Read the model definition and answer for the solid it produces. Units are mm, in the model's axes. A direction names the side the tool comes from. Coordinates: 2 decimals unless noted, no trailing zeros. Write each loop counter-clockwise with the first axis right and the second up, starting at its lowest first coordinate (ties: lowest second). Pieces come first, ordered by that corner, then holes. Notation, with made-up numbers: (34, 85) -> (39, 85) arc R32 ccw to (39, 116) -> close; hole circle Ø1 at (33, 86). An arc over 180 degrees is marked (long way). Use CSV: the item, a comma, the result in double quotes.
Autodesk Inventor part; units mm, degrees
ref_plane "YZ Plane" through (0, 0, 0) normal (1, 0, 0) x (0, 1, 0)
ref_plane "XZ Plane" through (0, 0, 0) normal (0, 1, 0) x (-1, 0, 0)
ref_plane "XY Plane" through (0, 0, 0) normal (0, 0, 1) x (1, 0, 0)
sketch "Sketch1" plane through (0, 0, 0) normal (0, 0, 1) x (1, 0, 0)
  circle A0 centre (0, 0) radius 22.225
  circle A1 centre (0, 0) radius 28.575
  line L0 (0, 0) -> (-22.225, 0) construction
  line L1 (-26.1937, 1.5875) -> (-24.6062, 1.5875)
  line L2 (-24.6062, 1.5875) -> (-24.6062, -1.5875)
  line L3 (-24.6062, -1.5875) -> (-26.1937, -1.5875)
  line L4 (-26.1937, -1.5875) -> (-26.1937, 1.5875)
  line L5 (-22.225, 0) -> (-28.575, 0) construction
  line L6 (-25.4, 1.5875) -> (-25.4, -1.5875) construction
  line L7 (-23.4782, -11.7221) -> (-22.1034, -10.9283)
  line L8 (-22.1034, -10.9283) -> (-20.5159, -13.6779)
  line L9 (-20.5159, -13.6779) -> (-21.8907, -14.4717)
  line L10 (-21.8907, -14.4717) -> (-23.4782, -11.7221)
  line L11 (-22.7908, -11.3252) -> (-21.2033, -14.0748) construction
  line L12 (-14.4717, -21.8907) -> (-13.6779, -20.5159)
  line L13 (-13.6779, -20.5159) -> (-10.9283, -22.1034)
  line L14 (-10.9283, -22.1034) -> (-11.7221, -23.4782)
  line L15 (-11.7221, -23.4782) -> (-14.4717, -21.8907)
  line L16 (-14.0748, -21.2033) -> (-11.3252, -22.7908) construction
  line L17 (-1.5875, -26.1938) -> (-1.5875, -24.6063)
  line L18 (-1.5875, -24.6063) -> (1.5875, -24.6063)
  line L19 (1.5875, -24.6063) -> (1.5875, -26.1938)
  line L20 (1.5875, -26.1938) -> (-1.5875, -26.1938)
  line L21 (-1.5875, -25.4) -> (1.5875, -25.4) construction
  line L22 (11.7221, -23.4782) -> (10.9283, -22.1034)
  line L23 (10.9283, -22.1034) -> (13.6779, -20.5159)
  line L24 (13.6779, -20.5159) -> (14.4717, -21.8907)
  line L25 (14.4717, -21.8907) -> (11.7221, -23.4782)
  line L26 (11.3252, -22.7908) -> (14.0748, -21.2033) construction
  line L27 (21.8907, -14.4717) -> (20.5159, -13.6779)
  line L28 (20.5159, -13.6779) -> (22.1034, -10.9283)
  line L29 (22.1034, -10.9283) -> (23.4782, -11.7221)
  line L30 (23.4782, -11.7221) -> (21.8907, -14.4717)
  line L31 (21.2033, -14.0748) -> (22.7908, -11.3252) construction
  line L32 (26.1938, -1.5875) -> (24.6063, -1.5875)
  line L33 (24.6063, -1.5875) -> (24.6063, 1.5875)
  line L34 (24.6063, 1.5875) -> (26.1938, 1.5875)
  line L35 (26.1938, 1.5875) -> (26.1938, -1.5875)
  line L36 (25.4, -1.5875) -> (25.4, 1.5875) construction
  line L37 (23.4782, 11.7221) -> (22.1034, 10.9283)
  line L38 (22.1034, 10.9283) -> (20.5159, 13.6779)
  line L39 (20.5159, 13.6779) -> (21.8907, 14.4717)
  line L40 (21.8907, 14.4717) -> (23.4782, 11.7221)
  line L41 (22.7908, 11.3252) -> (21.2033, 14.0748) construction
  line L42 (14.4717, 21.8907) -> (13.6779, 20.5159)
  line L43 (13.6779, 20.5159) -> (10.9283, 22.1034)
  line L44 (10.9283, 22.1034) -> (11.7221, 23.4782)
  line L45 (11.7221, 23.4782) -> (14.4717, 21.8907)
  line L46 (14.0748, 21.2033) -> (11.3252, 22.7908) construction
  line L47 (1.5875, 26.1937) -> (1.5875, 24.6063)
  line L48 (1.5875, 24.6063) -> (-1.5875, 24.6063)
  line L49 (-1.5875, 24.6063) -> (-1.5875, 26.1938)
  line L50 (-1.5875, 26.1938) -> (1.5875, 26.1937)
  line L51 (1.5875, 25.4) -> (-1.5875, 25.4) construction
  line L52 (-11.7221, 23.4782) -> (-10.9283, 22.1034)
  line L53 (-10.9283, 22.1034) -> (-13.6779, 20.5159)
  line L54 (-13.6779, 20.5159) -> (-14.4717, 21.8907)
  line L55 (-14.4717, 21.8907) -> (-11.7221, 23.4782)
  line L56 (-11.3252, 22.7908) -> (-14.0748, 21.2033) construction
  line L57 (-21.8907, 14.4717) -> (-20.5159, 13.6779)
  line L58 (-20.5159, 13.6779) -> (-22.1034, 10.9283)
  line L59 (-22.1034, 10.9283) -> (-23.4782, 11.7221)
  line L60 (-23.4782, 11.7221) -> (-21.8907, 14.4717)
  line L61 (-21.2033, 14.0748) -> (-22.7908, 11.3252) construction
  point P0 (-26.1937, 0)
  point P1 (-25.4, 0)
  point P2 (-22.6845, -13.0969)
  point P3 (-21.997, -12.7)
  point P4 (-13.0969, -22.6845)
  point P5 (-12.7, -21.997)
  point P6 (0, -26.1937)
  point P7 (0, -25.4)
  point P8 (13.0969, -22.6845)
  point P9 (12.7, -21.997)
  point P10 (22.6845, -13.0969)
  point P11 (21.997, -12.7)
  point P12 (26.1937, 0)
  point P13 (25.4, 0)
  point P14 (22.6845, 13.0969)
  point P15 (21.997, 12.7)
  point P16 (13.0969, 22.6845)
  point P17 (12.7, 21.997)
  point P18 (0, 26.1937)
  point P19 (0, 25.4)
  point P20 (-13.0969, 22.6845)
  point P21 (-12.7, 21.997)
  point P22 (-22.6845, 13.0969)
  point P23 (-21.997, 12.7)
  dimension "d0" = 44.45
  dimension "d1" = 57.15
  dimension "d2" = 3.175
  dimension "d3" = 1.5875
  dimension "d6" = 360
extrude "Extrusion1" add sketch "Sketch1" against normal blind 1.5875 contours A1 | L1 L2 L3 L4 | L7 L8 L9 L10 | L12 L13 L14 L15 | L17 L18 L19 L20 | L22 L23 L24 L25 | L27 L28 L29 L30 | L32 L33 L34 L35 | L37 L38 L39 L40 | L42 L43 L44 L45 | L47 L48 L49 L50 | L52 L53 L54 L55 | L57 L58 L59 L60
extrude "Extrusion2" add sketch "Sketch1" along normal blind 1.27 contours L1 L2 L3 L4 | L7 L8 L9 L10 | L12 L13 L14 L15 | L17 L18 L19 L20 | L22 L23 L24 L25 | L27 L28 L29 L30 | L32 L33 L34 L35 | L37 L38 L39 L40 | L42 L43 L44 L45 | L47 L48 L49 L50 | L52 L53 L54 L55 | L57 L58 L59 L60
properties part number "LED Ring"
1. Find the intervals of material crossed by line 1 along Y through (x, z) = (0, -0.55) (3 decimals); line 2 along X through (y, z) = (1, 1); line 3 along Y through (x, z) = (19, -0.05), in increasing order.
Solutions:
line 1,"y = -28.575 to -22.225, 22.225 to 28.575"
line 2,"x = -26.19 to -24.61, 24.61 to 26.19"
line 3,"y = -21.34 to -11.53, 11.53 to 21.34"
2. A cutting plane is placed at B-B (x = 3.5). Give the vertices of the cut face in (y, z).
Solutions:
outline,"(-28.36, -1.59) -> (-21.95, -1.59) -> (-21.95, 0) -> (-28.36, 0) -> close; (21.95, -1.59) -> (28.36, -1.59) -> (28.36, 0) -> (21.95, 0) -> close"
3. A cutting plane is placed at C-C (y = -18). Give the vertices of the cut face in (x, z), and give its area (3 significant figures).
Solutions:
outline,"(-22.19, -1.59) -> (-13.04, -1.59) -> (-13.04, 0) -> (-22.19, 0) -> close; (13.04, -1.59) -> (22.19, -1.59) -> (22.19, 0) -> (13.04, 0) -> close"
area,"29.1 mm^2"
4. Each of these flat-tipped pins is pushed along its axis until it touches: pin 1 Ø0.6 at (x, z) = (1, 0.5) entering from -Y; pin 2 Ø0.6 at (y, z) = (-0.5, 0.5) entering from +X; pin 3 Ø0.6 at (x, z) = (-25, 0.5) entering from +Y. Where does it stop, or does it pass through?
Solutions:
pin 1,"stops at y = -26.19"
pin 2,"stops at x = 26.19"
pin 3,"stops at y = 1.59"
5. A cutting plane is placed at A-A (y = 0). Give the vertices of the cut face in (x, z) (1 decimal), and give its area (3 significant figures).
Solutions:
outline,"(-28.6, -1.6) -> (-22.2, -1.6) -> (-22.2, 0) -> (-24.6, 0) -> (-24.6, 1.3) -> (-26.2, 1.3) -> (-26.2, 0) -> (-28.6, 0) -> close; (22.2, -1.6) -> (28.6, -1.6) -> (28.6, 0) -> (26.2, 0) -> (26.2, 1.3) -> (24.6, 1.3) -> (24.6, 0) -> (22.2, 0) -> close"
area,"24.2 mm^2"
6. A tool of negligible diameter and unlimited length cuts with its end or side. For faces 4 (the flat face through (25, -1.588, 1)), 5 (the flat face through (13.12, -22.67, 0.63)), 6 (the flat face through (1.588, 25, 1)), 7 (the flat face through (24.606, 0, 1)), 8 (the flat face through (13.078, 22.696, 0.626)), from which of +Z, -Z, +X, -X, +Y, -Y can it reach the whole face along a straight path? Write none if from no direction.
Solutions:
face 4,"+Z, +X, -X, -Y"
face 5,"+Z, +X, -Y"
face 6,"+Z, +X, +Y, -Y"
face 7,"+Z, +Y, -Y"
face 8,"+Z, +X, +Y"
7. For a pull along X with two mould halves and no side action, classify faces 1 (the flat face through (-1.588, -25, 1)), 2 (the flat face through (-21.21, 14.08, 0.63)), 3 (the flat face through (0, -26.194, 1)) as pulls with the +X half, pulls with the -X half, needs draft (parallel to the pull), parting line crosses it, or undercut.
Solutions:
face 1,"pulls with the -X half"
face 2,"undercut"
face 3,"needs draft"
